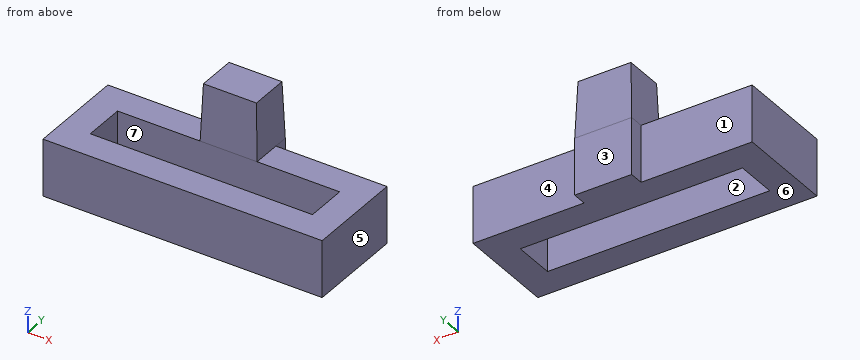
```python
from build123d import *

# Parameters (mm, degrees)
ESQUISSE1_W        = 19.6
ESQUISSE1_H        = 6.9
ESQUISSE1_W_2      = 15.6
ESQUISSE1_H_2      = 2.9
EXTRU_MINCE1_DEPTH = 4
ESQUISSE2_W        = 4
ESQUISSE2_H        = 3
BOSS_EXTRU_2_DEPTH = 4
ESQUISSE3_W        = 4
ESQUISSE3_H        = 3
BOSS_EXTRU_3_DEPTH = 4
BOSS_EXTRU_3_TAPER = 2


with BuildPart() as part:
    # Esquisse1 → Extru.-Mince1 (new body)
    with BuildSketch(Plane.XY):
        with Locations((7.8, 1.45)):
            Rectangle(ESQUISSE1_W, ESQUISSE1_H)
        with Locations((7.8, 1.45)):
            Rectangle(ESQUISSE1_W_2, ESQUISSE1_H_2, mode=Mode.SUBTRACT)
    extrude(amount=EXTRU_MINCE1_DEPTH)

    # Esquisse2 → Boss.-Extru.2 (add)
    with BuildSketch(Plane.XY):
        with Locations((7.8, 4.4)):
            Rectangle(ESQUISSE2_W, ESQUISSE2_H)
    extrude(amount=BOSS_EXTRU_2_DEPTH)

    # Esquisse3 → Boss.-Extru.3 (add)
    with BuildSketch(Plane.XY.offset(4)):
        with Locations((7.8, 4.4)):
            Rectangle(ESQUISSE3_W, ESQUISSE3_H)
    extrude(amount=BOSS_EXTRU_3_DEPTH, taper=BOSS_EXTRU_3_TAPER)


solid = part.part
```
Read the model definition and answer for the solid it produces. Units are mm, in the model's axes. Face numbers are marked on the shaded views. A direction names the side the tool comes from. Coordinates: 2 decimals unless noted, no trailing zeros. Loops run counter-clockwise (first coordinate to the right, second up) from the corner with the lowest first, then second, coordinate; pieces in that order, holes last. Notation, with made-up numbers: (69.25, 16) - (77.25, 16) arc R22 cw to (77.25, 55) - close; hole circle Ø8 at (-19.75, 17). An arc over 180 degrees is marked (long way). Answer in a Markdown table with one row per item.
1. Given pin 1 (3.5 mm diameter, centred on x = 6.5, y = 1, fed in from +Z); pin 2 (0.5 mm diameter, centred on y = 5.5, z = 2.5, fed in from +X); pin 3 (0.8 mm diameter, centred on y = 5.5, z = 1.5, fed in from -X), each flat-ended and moving along its own axis, determine where each tip first touches the part or whether it passes through.
Conclusion:
| item | result |
|---|---|
| pin 1 | stops at z = 4 |
| pin 2 | stops at x = 9.8 |
| pin 3 | stops at x = 5.8 |
2. Find section C-C, the plane z = 1.25. Write down the section's boundary in (x, y).
Conclusion:
| item | result |
|---|---|
| outline | (-2, -2) - (17.6, -2) - (17.6, 4.9) - (9.8, 4.9) - (9.8, 5.9) - (5.8, 5.9) - (5.8, 4.9) - (-2, 4.9) - close; hole (0, 0) - (15.6, 0) - (15.6, 2.9) - (0, 2.9) - close |
3. Find section D-D, the plane y = 5.25. Write down the section's boundary in (x, z), then the cut area to 3 significant figures.
Conclusion:
| item | result |
|---|---|
| outline | (5.8, 0) - (9.8, 0) - (9.8, 4) - (9.66, 8) - (5.94, 8) - (5.8, 4) - close |
| area | 31.4 mm² |
4. Find section B-B, the plane y = 2.5. Write down the section's boundary in (x, z).
Conclusion:
| item | result |
|---|---|
| outline | (-2, 0) - (0, 0) - (0, 4) - (-2, 4) - close; (15.6, 0) - (17.6, 0) - (17.6, 4) - (15.6, 4) - close |
5. Which of the six approach directions +Z, -Z, +X, -X, +Y, -Y give full straight-line access (tool end or side, diameter ignored) to the marked faces 1, 2, 3 and 4?
Conclusion:
| item | result |
|---|---|
| face 1 | +Z, -Z, -X, +Y |
| face 2 | +Z, -Z |
| face 3 | +Z, -Z, +X, -X, +Y |
| face 4 | +Z, -Z, +X, +Y |
6. Straight lines are drawn through the part: line 1 (Y direction, x = 7, z = 2); line 2 (Y direction, x = 12.5, z = 1.5); line 3 (X direction, y = 2.75, z = 1.75). For each, find the intervals that lie inside material, in ascending order.
Conclusion:
| item | result |
|---|---|
| line 1 | y = -2 to 0, 2.9 to 5.9 |
| line 2 | y = -2 to 0, 2.9 to 4.9 |
| line 3 | x = -2 to 0, 15.6 to 17.6 |
7. Find section A-A, the plane x = 7.75. Write down the section's boundary in (y, z).
Conclusion:
| item | result |
|---|---|
| outline | (-2, 0) - (0, 0) - (0, 4) - (-2, 4) - close; (2.9, 0) - (5.9, 0) - (5.9, 4) - (5.76, 8) - (3.04, 8) - (2.9, 4) - close |
8. Determine the mould class of the marked faces 5, 6 and 7 for opening direction X: +X half, -X half, draft (parallel to the pull), parting line (faces both ways), or undercut.
Conclusion:
| item | result |
|---|---|
| face 5 | +X half |
| face 6 | draft |
| face 7 | undercut |
